from build123d import *

# Parameters (mm, degrees)
IZIM1_R                          = 37
IZIM1_R_2                        = 35.75
Y_KSEKLIK_EKSTR_ZYON5_DEPTH      = 5
Y_KSEKLIK_EKSTR_ZYON5_DEPTH_BACK = 5
IZIM1_13_R                       = 38.25
IZIM1_13_R_2                     = 37
Y_KSEKLIK_EKSTR_ZYON6_DEPTH      = 3
Y_KSEKLIK_EKSTR_ZYON6_DEPTH_BACK = 3
IZIM1_14_R                       = 1.5
Y_KSEKLIK_EKSTR_ZYON7_DEPTH      = 3
Y_KSEKLIK_EKSTR_ZYON7_DEPTH_BACK = 3
Y_KSEKLIK_EKSTR_ZYON8_DEPTH      = 7
Y_KSEKLIK_EKSTR_ZYON8_DEPTH_BACK = 3


with BuildPart() as part:
    # izim1 → Y_kseklik-Ekstr_zyon5 (new body, two sides)
    with BuildSketch(Plane.XY) as y_kseklik_ekstr_zyon5_sk:
        Circle(IZIM1_R)
        Circle(IZIM1_R_2, mode=Mode.SUBTRACT)
    extrude(amount=Y_KSEKLIK_EKSTR_ZYON5_DEPTH)
    extrude(y_kseklik_ekstr_zyon5_sk.sketch, amount=-Y_KSEKLIK_EKSTR_ZYON5_DEPTH_BACK)

    # izim1_13 → Y_kseklik-Ekstr_zyon6 (add, two sides)
    with BuildSketch(Plane.XY) as y_kseklik_ekstr_zyon6_sk:
        Circle(IZIM1_13_R)
        Circle(IZIM1_13_R_2, mode=Mode.SUBTRACT)
    extrude(amount=Y_KSEKLIK_EKSTR_ZYON6_DEPTH)
    extrude(y_kseklik_ekstr_zyon6_sk.sketch, amount=-Y_KSEKLIK_EKSTR_ZYON6_DEPTH_BACK)

    # izim1_14 → Y_kseklik-Ekstr_zyon7 (add, two sides)
    with BuildSketch(Plane.XY) as y_kseklik_ekstr_zyon7_sk:
        with BuildLine():
            Line((0.345332455, 10.619791473), (0.345332455, 8.211364581))
            Line((0.345332455, 8.211364581), (0.345332455, 2.892483792))
            ThreePointArc((0.345332455, 2.892483792), (2.178494802, 1.93387626), (2.913025402, 0))
            ThreePointArc((2.913025402, 0), (-1.934432099, -2.17800125), (-0.343856219, 2.892659657))
            Line((-0.343856219, 2.892659657), (-0.341141708, 8.211536302))
            Line((-0.341141708, 8.211536302), (-0.339912555, 10.619966332))
            ThreePointArc((-0.339912555, 10.619966332), (-1.789622614, 11.029720322), (-2.984950797, 11.946643504))
            Line((-2.984950797, 11.946643504), (-14.607897055, 30.387938553))
            Line((-14.607897055, 30.387938553), (-14.847878363, 30.848411366))
            ThreePointArc((-14.847878363, 30.848411366), (-14.740281438, 32.044676397), (-13.92488883, 32.926584565))
            ThreePointArc((-13.92488883, 32.926584565), (-17.875, 30.960408185), (-21.552814278, 28.522599754))
            ThreePointArc((-21.552814278, 28.522599754), (-20.401800041, 28.78442387), (-19.324525803, 28.301862102))
            Line((-19.324525803, 28.301862102), (-19.045735303, 27.863795787))
            Line((-19.045735303, 27.863795787), (-8.886868167, 8.577081355))
            ThreePointArc((-8.886868167, 8.577081355), (-9.303777514, 5.496482546), (-11.800782256, 3.644761794))
            Line((-11.800782256, 3.644761794), (-33.653555768, 2.549643924))
            Line((-33.653555768, 2.549643924), (-34.19029782, 2.590308308))
            ThreePointArc((-34.19029782, 2.590308308), (-35.134400226, 3.283913251), (-35.477703108, 4.403984811))
            ThreePointArc((-35.477703108, 4.403984811), (-35.75, 0), (-35.477703108, -4.403984811))
            ThreePointArc((-35.477703108, -4.403984811), (-35.134400226, -3.283913251), (-34.19029782, -2.590308308))
            Line((-34.19029782, -2.590308308), (-33.653555768, -2.549643924))
            Line((-33.653555768, -2.549643924), (-11.802585687, -3.638917628))
            ThreePointArc((-11.802585687, -3.638917628), (-9.303458853, -5.492132995), (-8.888309481, -8.575587733))
            Line((-8.888309481, -8.575587733), (-19.045735303, -27.863795787))
            ThreePointArc((-19.045735303, -27.863795787), (-20.165883221, -28.700819486), (-21.552814278, -28.522599754))
            ThreePointArc((-21.552814278, -28.522599754), (-17.875, -30.960408185), (-13.92488883, -32.926584565))
            ThreePointArc((-13.92488883, -32.926584565), (-14.772697173, -31.814576902), (-14.607887345, -30.4259885))
            Line((-14.607887345, -30.4259885), (-2.984941087, -11.98469345))
            ThreePointArc((-2.984941087, -11.98469345), (0.002715908, -10.643228062), (2.991057136, -11.983168513))
            Line((2.991057136, -11.983168513), (14.663708375, -30.397995932))
            ThreePointArc((14.663708375, -30.397995932), (14.817986455, -31.815304786), (13.92488883, -32.926584565))
            ThreePointArc((13.92488883, -32.926584565), (17.875, -30.960408185), (21.552814278, -28.522599754))
            ThreePointArc((21.552814278, -28.522599754), (20.242255546, -28.76161283), (19.107217792, -28.064202809))
            Line((19.107217792, -28.064202809), (18.993975038, -27.89787469))
            Line((18.993975038, -27.89787469), (8.881942007, -8.582182507))
            ThreePointArc((8.881942007, -8.582182507), (9.294710999, -5.488602486), (11.804336715, -3.633233425))
            Line((11.804336715, -3.633233425), (33.657290889, -2.499854))
            Line((33.657290889, -2.499854), (33.849149755, -2.514104082))
            ThreePointArc((33.849149755, -2.514104082), (35.026532395, -3.146147751), (35.477703108, -4.403984811))
            ThreePointArc((35.477703108, -4.403984811), (35.681860841, -2.206197397), (35.75, 0))
            ThreePointArc((35.75, 0), (35.681860841, 2.206197397), (35.477703108, 4.403984811))
            ThreePointArc((35.477703108, 4.403984811), (35.026532395, 3.146147751), (33.849149755, 2.514104082))
            Line((33.849149755, 2.514104082), (33.657290889, 2.499854))
            Line((33.657290889, 2.499854), (11.803877394, 3.634725418))
            ThreePointArc((11.803877394, 3.634725418), (9.295867667, 5.489285508), (8.88302669, 8.581059795))
            Line((8.88302669, 8.581059795), (18.993975038, 27.89787469))
            Line((18.993975038, 27.89787469), (18.993582514, 27.898141932))
            ThreePointArc((18.993582514, 27.898141932), (20.143868947, 28.740405096), (21.552814278, 28.522599754))
            ThreePointArc((21.552814278, 28.522599754), (17.875, 30.960408185), (13.92488883, 32.926584565))
            ThreePointArc((13.92488883, 32.926584565), (14.836394127, 31.799309486), (14.663698665, 30.359945986))
            Line((14.663698665, 30.359945986), (14.663270965, 30.360152301))
            Line((14.663270965, 30.360152301), (2.991047427, 11.945118566))
            ThreePointArc((2.991047427, 11.945118566), (1.795251444, 11.028805544), (0.345332455, 10.619791473))
        make_face()
        with BuildLine():
            ThreePointArc((-15.330091906, -28.374268836), (-15.633406502, -28.599064993), (-16.007432074, -28.547704226))
            Line((-16.007432074, -28.547704226), (-16.719321042, -28.136694938))
            ThreePointArc((-16.719321042, -28.136694938), (-16.950813558, -27.838459675), (-16.907791673, -27.46338345))
            Line((-16.907791673, -27.46338345), (-8.752791972, -12.583042517))
            ThreePointArc((-8.752791972, -12.583042517), (-8.44909878, -12.341848787), (-8.064321341, -12.3903286))
            Line((-8.064321341, -12.3903286), (-6.698178659, -13.179071446))
            ThreePointArc((-6.698178659, -13.179071446), (-6.463805189, -13.488058576), (-6.52083849, -13.87166146))
            Line((-6.52083849, -13.87166146), (-15.330091906, -28.374268836))
        make_face(mode=Mode.SUBTRACT)
        with Locations((-4.7625, -8.25)):
            Circle(IZIM1_14_R, mode=Mode.SUBTRACT)
        with BuildLine():
            Line((16.719321042, -28.136694938), (16.007432074, -28.547704226))
            ThreePointArc((16.007432074, -28.547704226), (15.633406502, -28.599064993), (15.330091906, -28.374268836))
            Line((15.330091906, -28.374268836), (6.52083849, -13.87166146))
            ThreePointArc((6.52083849, -13.87166146), (6.463805189, -13.488058576), (6.698178659, -13.179071446))
            Line((6.698178659, -13.179071446), (8.064321341, -12.3903286))
            ThreePointArc((8.064321341, -12.3903286), (8.44909878, -12.341848787), (8.752791972, -12.583042517))
            Line((8.752791972, -12.583042517), (16.907791673, -27.46338345))
            ThreePointArc((16.907791673, -27.46338345), (16.950813558, -27.838459675), (16.719321042, -28.136694938))
        make_face(mode=Mode.SUBTRACT)
        with Locations((4.7625, -8.25)):
            Circle(IZIM1_14_R, mode=Mode.SUBTRACT)
        with BuildLine():
            Line((-32.726753116, -0.411009288), (-32.726753116, 0.411009288))
            ThreePointArc((-32.726753116, 0.411009288), (-32.584220059, 0.760605318), (-32.237883578, 0.910885385))
            Line((-32.237883578, 0.910885385), (-15.273630462, 1.288618943))
            ThreePointArc((-15.273630462, 1.288618943), (-14.91290397, 1.146209789), (-14.7625, 0.788742846))
            Line((-14.7625, 0.788742846), (-14.7625, -0.788742846))
            ThreePointArc((-14.7625, -0.788742846), (-14.91290397, -1.146209789), (-15.273630462, -1.288618943))
            Line((-15.273630462, -1.288618943), (-32.237883578, -0.910885385))
            ThreePointArc((-32.237883578, -0.910885385), (-32.584220059, -0.760605318), (-32.726753116, -0.411009288))
        make_face(mode=Mode.SUBTRACT)
        with Locations((-4.7625, 0)):
            Circle(IZIM1_14_R, mode=Mode.SUBTRACT)
        with Locations((-4.7625, 8.25)):
            Circle(IZIM1_14_R, mode=Mode.SUBTRACT)
        with BuildLine():
            ThreePointArc((-6.52083849, 13.87166146), (-6.463805189, 13.488058576), (-6.698178659, 13.179071446))
            Line((-6.698178659, 13.179071446), (-8.064321341, 12.3903286))
            ThreePointArc((-8.064321341, 12.3903286), (-8.44909878, 12.341848787), (-8.752791972, 12.583042517))
            Line((-8.752791972, 12.583042517), (-16.907791673, 27.46338345))
            ThreePointArc((-16.907791673, 27.46338345), (-16.950813558, 27.838459675), (-16.719321042, 28.136694938))
            Line((-16.719321042, 28.136694938), (-16.007432074, 28.547704226))
            ThreePointArc((-16.007432074, 28.547704226), (-15.633406502, 28.599064993), (-15.330091906, 28.374268836))
            Line((-15.330091906, 28.374268836), (-6.52083849, 13.87166146))
        make_face(mode=Mode.SUBTRACT)
        with Locations((4.7625, 0)):
            Circle(IZIM1_14_R, mode=Mode.SUBTRACT)
        with Locations((4.7625, 8.25)):
            Circle(IZIM1_14_R, mode=Mode.SUBTRACT)
        with BuildLine():
            ThreePointArc((32.237883578, 0.910885385), (32.584220059, 0.760605318), (32.726753116, 0.411009288))
            Line((32.726753116, 0.411009288), (32.726753116, -0.411009288))
            ThreePointArc((32.726753116, -0.411009288), (32.584220059, -0.760605318), (32.237883578, -0.910885385))
            Line((32.237883578, -0.910885385), (15.273630462, -1.288618943))
            ThreePointArc((15.273630462, -1.288618943), (14.91290397, -1.146209789), (14.7625, -0.788742846))
            Line((14.7625, -0.788742846), (14.7625, 0.788742846))
            ThreePointArc((14.7625, 0.788742846), (14.91290397, 1.146209789), (15.273630462, 1.288618943))
            Line((15.273630462, 1.288618943), (32.237883578, 0.910885385))
        make_face(mode=Mode.SUBTRACT)
        with BuildLine():
            Line((8.064321341, 12.3903286), (6.698178659, 13.179071446))
            ThreePointArc((6.698178659, 13.179071446), (6.463805189, 13.488058576), (6.52083849, 13.87166146))
            Line((6.52083849, 13.87166146), (15.330091906, 28.374268836))
            ThreePointArc((15.330091906, 28.374268836), (15.633406502, 28.599064993), (16.007432074, 28.547704226))
            Line((16.007432074, 28.547704226), (16.719321042, 28.136694938))
            ThreePointArc((16.719321042, 28.136694938), (16.950813558, 27.838459675), (16.907791673, 27.46338345))
            Line((16.907791673, 27.46338345), (8.752791972, 12.583042517))
            ThreePointArc((8.752791972, 12.583042517), (8.44909878, 12.341848787), (8.064321341, 12.3903286))
        make_face(mode=Mode.SUBTRACT)
    extrude(amount=Y_KSEKLIK_EKSTR_ZYON7_DEPTH)
    extrude(y_kseklik_ekstr_zyon7_sk.sketch, amount=-Y_KSEKLIK_EKSTR_ZYON7_DEPTH_BACK)

    # izim1_17 → Y_kseklik-Ekstr_zyon8 (add, two sides)
    with BuildSketch(Plane.XY) as y_kseklik_ekstr_zyon8_sk:
        with BuildLine():
            ThreePointArc((2.913025402, 0), (2.178494802, 1.93387626), (0.345332455, 2.892483792))
            Line((0.345332455, 2.892483792), (0.345332455, 1.969960785))
            ThreePointArc((0.345332455, 1.969960785), (1.794746568, 0.882544479), (1.770998825, -0.929280992))
            Line((1.770998825, -0.929280992), (-1.770998825, -0.929280992))
            ThreePointArc((-1.770998825, -0.929280992), (-1.794521304, 0.883002429), (-0.344327032, 1.970136771))
            Line((-0.344327032, 1.970136771), (-0.343856219, 2.892659657))
            ThreePointArc((-0.343856219, 2.892659657), (-1.934432099, -2.17800125), (2.913025402, 0))
        make_face()
    extrude(amount=Y_KSEKLIK_EKSTR_ZYON8_DEPTH)
    extrude(y_kseklik_ekstr_zyon8_sk.sketch, amount=-Y_KSEKLIK_EKSTR_ZYON8_DEPTH_BACK)


solid = part.part
Can you work these out from the model? Positions are in its coordinate system, mm. A direction names the side the tool comes from. Coordinates: 2 decimals unless noted, no trailing zeros. Put each result on its own line as item: value. Start each with the question number.
Item 1: If we mould it in two halves opening along Y, with no side actions, what happens to faces 1 (the face through (0, -0.929, 2)), 2 (the face through (-19.4, 30.3, -5))? For each: +Y half, -Y half, draft (parallel to the pull), parting line (faces both ways), or undercut.
Item 2: Suppose I cut it at A-A (y = -18). State how many separate pieces and enclosed holes the cut face has, and give its area (3 significant figures).
Item 3: Which directions (+Z, -Z, +X, -X, +Y, -Y) give clear straight access to the entire face, cutting with the end or side of a thin tool? Please do faces 3 (the face through (0, -1.3, 7)), 4 (the face through (-13.896, -18.085, 0.042)).
Item 4: For pin 1 (3 mm diameter, centred on y = -2, z = 2.5, fed in from +X); pin 2 (4 mm diameter, centred on x = 21.5, y = 2, fed in from +Z); pin 3 (3.5 mm diameter, centred on x = 4.76, y = 8.25, fed in from -Z), each with a flat end and sliding along its axis, tell me the tip position at first contact or that it passes through.
Item 5: If I drill on line 1 along X through (y, z) = (23, -2); line 2 along Y through (x, z) = (-25.5, 0.25); line 3 along Y through (x, z) = (-23.5, -2), over which ranges is the centre line in solid material (lowest first)?
Here are the results:
1. face 1: undercut
1. face 2: draft
2. separate pieces: 6
2. enclosed holes: 0
2. area: 98.0 mm²
3. face 3: +Z, +X, -X, +Y, -Y
3. face 4: +Z, -Z
4. pin 1: x = 38.25
4. pin 2: z = 3
4. pin 3: z = -3
5. line 1: -30.56 to -27.37, -16.48 to -14.46, -12.07 to -9.95, 10 to 12.07, 14.46 to 16.43, 27.37 to 30.56
5. line 2: -28.51 to -25.06, -2.96 to -1.06, 1.06 to 2.96, 25.06 to 28.51
5. line 3: -30.18 to -26.94, -3.06 to -1.11, 1.11 to 3.06, 26.94 to 30.18
